```python
from build123d import *

# Parameters (mm, degrees)
BODY_KEY_DEPTH      = 9.9375
BOSS_EXTRUDE1_DEPTH = 27.16


with BuildPart() as part:
    # Sketch3 → Body (revolve)
    with BuildSketch(Plane(origin=(0, 0, 0), x_dir=(0, 0, -1), z_dir=(1, 0, 0)), mode=Mode.PRIVATE) as body_sk:
        Polygon((-31.75, 0), (68.625, 0), (68.625, 7.9375), (-30.350404591, 7.9375), (-31.75, 6.537904591), align=None)
    revolve(body_sk.sketch.rotate(Axis((0, 0, -80.9), (0, 0, 1)), 90), axis=Axis((0, 0, -80.9), (0, 0, 1)))

    # Sketch4 → Body-Back (revolve)
    with BuildSketch(Plane(origin=(0, 0, 0), x_dir=(0, 0, -1), z_dir=(1, 0, 0)), mode=Mode.PRIVATE) as body_back_sk:
        Polygon((68.625, 0), (68.625, 2.5), (168.330127019, 2.5), (169, 1.830127019), (169, 0), align=None)
    revolve(body_back_sk.sketch.rotate(Axis((0, 0, -80.9), (0, 0, 1)), 90), axis=Axis((0, 0, -80.9), (0, 0, 1)))

    # Sketch7 → Body-Key (add)
    with BuildSketch(Plane(origin=(0, 0, 0), x_dir=(1, 0, 0), z_dir=(0, 1, 0))):
        with BuildLine():
            Line((-2.5, -31.75), (2.5, -31.75))
            Line((2.5, -31.75), (2.5, -9.25))
            ThreePointArc((2.5, -9.25), (0, -6.75), (-2.5, -9.25))
            Line((-2.5, -9.25), (-2.5, -31.75))
        make_face()
    extrude(amount=BODY_KEY_DEPTH)

    # Sketch8 → Boss-Extrude1 (add)
    with BuildSketch(Plane.XY.offset(31.75)):
        with BuildLine():
            Line((2.5, 6.041042661), (2.5, 9.9375))
            Line((2.5, 9.9375), (-2.5, 9.9375))
            Line((-2.5, 9.9375), (-2.5, 6.041042661))
            ThreePointArc((-2.5, 6.041042661), (0, -6.537904591), (2.5, 6.041042661))
        make_face()
    extrude(amount=BOSS_EXTRUDE1_DEPTH)


solid = part.part
```
CAD build for the part. Positions are in the model's coordinates, mm. A direction names the side the tool comes from. Round coordinates to 2 decimals unless told otherwise and drop trailing zeros. Loops run counter-clockwise (first coordinate to the right, second up) from the corner with the lowest first, then second, coordinate; pieces in that order, holes last. Notation, with made-up numbers: M 19,75 L 28,75 A23 ccw 28,112 Z; hole C 85,-13.5 d2. An arc over 180 degrees is marked long. Return JSON: item names as keys, results as strings. Group by question number.
(1) Tool access for faces 1 (the flat face through (-2, -2, -68.625)), 2 (the flat face through (0, 9.938, 32)), 3 (the cylindrical face through (-0.252, -6.533, 45.14)), 4 (the flat face through (-2.5, 8, 34)), 5 (the flat face through (2.5, 8, 39)): list every direction of +Z, -Z, +X, -X, +Y, -Y with a clear straight run to the whole face (end or side of a thin tool).
(2) Wall check: probe 1 along Z at (x, y) = (6.5, 0) (3 decimals); probe 2 along X at (y, z) = (0.25, -20); probe 3 along Y at (x, z) = (4.5, -62.5). Give the ranges that are in metal, low to high. Write a range as [from, to].
(3) Saw through at C-C, the plane z = -21. List the corners of the cut face in (x, y) (1 decimal).
(4) Saw through at A-A, the plane z = -89. List the corners of the cut face in (x, y), and give its area (3 significant figures).
(5) Saw through at B-B, the plane z = 11.5. List the corners of the cut face in (x, y) (1 decimal), and give its area (3 significant figures).
(6) Drop flat-ended pins along their axis: P1, Ø3, axis at y = 8, z = 41, coming from the -X side; P2, Ø5, axis at y = -3.5, z = -137.5, coming from the -X side; P3, Ø5, axis at y = 3.5, z = -63.5, coming from the -X side. Give the stop position or say it passes through.
Answer list:
{
 "1": {"face 1": "-Z", "face 2": "+Z, -Z, +X, -X, +Y", "face 3": "+Z", "face 4": "+Z, -X, +Y", "face 5": "+Z, +X, +Y"},
 "2": {"probe 1": "[-68.625, 58.91]", "probe 2": "[-7.93, 7.93]", "probe 3": "[-6.54, 6.54]"},
 "3": {"outline": "C 0,0 d15.9"},
 "4": {"outline": "C 0,0 d5", "area": "19.6 mm2"},
 "5": {"outline": "M -2.5,7.5 A7.9 ccw long 2.5,7.5 L 2.5,9.9 L -2.5,9.9 Z", "area": "209 mm2"},
 "6": {"P1": "x = -2.5", "P2": "x = -2.29", "P3": "x = -7.87"}
}
